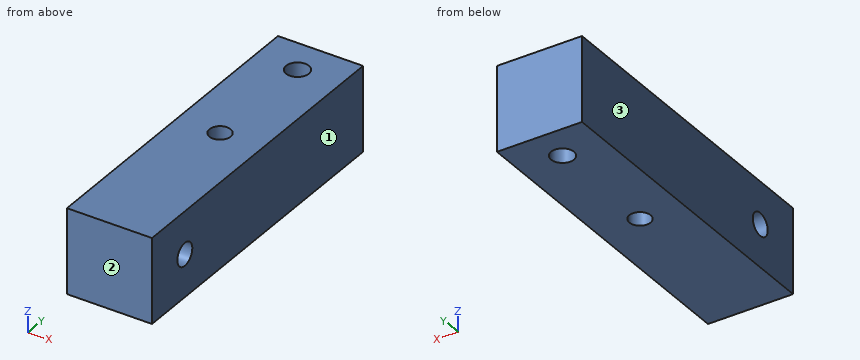
from build123d import *

# Parameters (mm, degrees)
SKETCH1_W           = 12.7
SKETCH1_H           = 12.7
BOSS_EXTRUDE1_DEPTH = 48.006
SKETCH2_R           = 1.5875
CUT_EXTRUDE1_DEPTH  = 51.061847109
SKETCH3_R           = 1.7
CUT_EXTRUDE2_DEPTH  = 51.061847109
SKETCH4_R           = 1.7
CUT_EXTRUDE3_DEPTH  = 51.061847109


with BuildPart() as part:
    # Sketch1 → Boss-Extrude1 (new body)
    with BuildSketch(Plane(origin=(0, 0, 0), x_dir=(1, 0, 0), z_dir=(0, 1, 0))):
        Rectangle(SKETCH1_W, SKETCH1_H)
    extrude(amount=BOSS_EXTRUDE1_DEPTH)

    # Sketch2 → Cut-Extrude1 (cut, through all)
    with BuildSketch(Plane.XY.offset(6.35)):
        with Locations((0, 25.146)):
            Circle(SKETCH2_R)
    extrude(amount=-CUT_EXTRUDE1_DEPTH, mode=Mode.SUBTRACT)

    # Sketch3 → Cut-Extrude2 (cut, through all)
    with BuildSketch(Plane.XY.offset(6.35)):
        with Locations((0, 42.76725)):
            Circle(SKETCH3_R)
    extrude(amount=-CUT_EXTRUDE2_DEPTH, mode=Mode.SUBTRACT)

    # Sketch4 → Cut-Extrude3 (cut, through all)
    with BuildSketch(Plane(origin=(6.35, 0, 0), x_dir=(0, 0, -1), z_dir=(1, 0, 0))):
        with Locations((0, 7.46125)):
            Circle(SKETCH4_R)
    extrude(amount=-CUT_EXTRUDE3_DEPTH, mode=Mode.SUBTRACT)


solid = part.part
Geometry check sheet. Reference: the model listing, model coordinates, mm. Face numbers are marked on the shaded views. Round coordinates to 2 decimals unless told otherwise and drop trailing zeros. Loops run counter-clockwise (first coordinate to the right, second up) from the corner with the lowest first, then second, coordinate; pieces in that order, holes last. Notation, with made-up numbers: (-26, -35.5) -> (31, -35.5) arc R19 cw to (31, -11.5) -> close; hole circle Ø3 at (46.25, 16.25). An arc over 180 degrees is marked (long way). Answer as a JSON object with one key per item and string values. Group by question number.
Item 1: Cross-section at B-B, the plane z = 0. Count the separate pieces of the cut face and the enclosed holes in it, plus the area to 4 significant figures.
Item 2: Depth check by flat-ended pin: pin 1 Ø2.5 at (x, y) = (0, 25.146) entering from +Z. Enter the tip coordinate at first touch or a pass-through.
Item 3: Release check for a two-part mould opening along X. For the marked faces 1, 2 and 3 record: pulls with the +X half, pulls with the -X half, needs draft (parallel to the pull), parting line crosses it, or undercut.
Item 4: Cross-section at A-A, the plane x = 0. Record the cut outline in (y, z).
Item 5: Thickness scan on line 1 along Y through (x, z) = (0, -2.5); line 2 along Y through (x, z) = (0, 0); line 3 along Y through (x, z) = (-2.5, 0). Record the ranges inside material, lowest first.
Determined:
{
 "1": {"separate pieces": "2", "enclosed holes": "2", "area": "549.5 mm²"},
 "2": {"pin 1": "passes through"},
 "3": {"face 1": "pulls with the +X half", "face 2": "needs draft", "face 3": "pulls with the -X half"},
 "4": {"outline": "(0, -6.35) -> (23.56, -6.35) -> (23.56, 6.35) -> (0, 6.35) -> close; (26.73, -6.35) -> (41.07, -6.35) -> (41.07, 6.35) -> (26.73, 6.35) -> close; (44.47, -6.35) -> (48.01, -6.35) -> (48.01, 6.35) -> (44.47, 6.35) -> close; hole circle Ø3.4 at (7.46, 0)"},
 "5": {"line 1": "y = 0 to 23.56, 26.73 to 41.07, 44.47 to 48.01", "line 2": "y = 0 to 5.76, 9.16 to 23.56, 26.73 to 41.07, 44.47 to 48.01", "line 3": "y = 0 to 5.76, 9.16 to 48.01"}
}
